```python
from build123d import *

# Parameters (mm, degrees)
SKETCH1_R               = 15
BOSS_EXTRUDE1_DEPTH     = 3.5
SKETCH2_R               = 2.121909517
SKETCH4_R               = 3.5
BOSS_EXTRUDE2_DEPTH     = 1
BOSS_EXTRUDE3_START     = 1
SKETCH5_R               = 3.5
BOSS_EXTRUDE3_DEPTH     = 1
CUT_EXTRUDE1_DEPTH      = 22.685248442
CUT_EXTRUDE1_DEPTH_BACK = 22.685248442
SKETCH3_R               = 2.5


with BuildPart() as part:
    # Sketch1 → Boss-Extrude1 (new body)
    with BuildSketch(Plane(origin=(0, 0, 0), x_dir=(1, 0, 0), z_dir=(0, 1, 0))):
        with Locations(Location((0, 0, 0), (0, 0, 270))):
            Circle(SKETCH1_R)
    extrude(amount=BOSS_EXTRUDE1_DEPTH)

    # Sketch2 → Cut-Revolve1 (revolve, cut)
    with BuildSketch(Plane(origin=(0, 0, 0), x_dir=(0, 0, -1), z_dir=(1, 0, 0)), mode=Mode.PRIVATE) as cut_revolve1_sk:
        with Locations((-16.2, 1.75)):
            Circle(SKETCH2_R)
    revolve(cut_revolve1_sk.sketch.rotate(Axis((0, 0, 0), (0, 1, 0)), 180), axis=Axis((0, 0, 0), (0, 1, 0)), mode=Mode.SUBTRACT)

    # Sketch4 → Boss-Extrude2 (add)
    with BuildSketch(Plane.XZ):
        with Locations(Location((0, 0, 0), (0, 0, 270))):
            Circle(SKETCH4_R)
    extrude(amount=BOSS_EXTRUDE2_DEPTH)

    # Sketch5 → Boss-Extrude3 (add)
    with BuildSketch(Plane(origin=(0, 3.5, 0), x_dir=(1, 0, 0), z_dir=(0, 1, 0)).offset(BOSS_EXTRUDE3_START)):
        with Locations(Location((0, 0, 0), (0, 0, 90))):
            Circle(SKETCH5_R)
    extrude(amount=-BOSS_EXTRUDE3_DEPTH)

    # Sketch3 → Cut-Extrude1 (cut, two sides: drawn at the far end of the back side and taken through both)
    with BuildSketch(Plane(origin=(0, 3.5, 0), x_dir=(1, 0, 0), z_dir=(0, 1, 0)).offset(-CUT_EXTRUDE1_DEPTH_BACK)):
        with Locations(Location((0, 0, 0), (0, 0, 270))):
            Circle(SKETCH3_R)
    extrude(amount=CUT_EXTRUDE1_DEPTH + CUT_EXTRUDE1_DEPTH_BACK, mode=Mode.SUBTRACT)


solid = part.part
```
Geometry check sheet. Reference: the model listing, model coordinates, mm. A direction names the side the tool comes from. Round coordinates to 2 decimals unless told otherwise and drop trailing zeros. Loops run counter-clockwise (first coordinate to the right, second up) from the corner with the lowest first, then second, coordinate; pieces in that order, holes last. Notation, with made-up numbers: (89.25, 15.25) - (143.25, 15.25) arc R34 cw to (143.25, 53.25) - close; hole circle Ø8 at (37.5, 30.5). An arc over 180 degrees is marked (long way). Write item = value, one per line. Start each with the question number.
1. Section check B-B on x = 0. Enter the section's corners in (y, z).
2. Set-up check for faces 1 (the face through (3.417, 4.007, 0.759)), 2 (the face through (-2, -1, -2)): record each of +Z, -Z, +X, -X, +Y, -Y from which the full face is reachable in a straight line by a thin tool's end or side.
3. Section check C-C on y = 0.45. Enter the section's corners in (x, z).
4. Thickness scan on line 1 (Y direction, x = 7.5, z = -11.5); line 2 (Z direction, x = 2, y = 0.2); line 3 (X direction, y = 1.1, z = 0). Record the ranges inside material, lowest first.
5. Depth check by flat-ended pin: pin 1 (3 mm diameter, centred on y = 1, z = 11, fed in from -X); pin 2 (6 mm diameter, centred on x = -5, z = -5, fed in from -Y); pin 3 (8 mm diameter, centred on x = 2.5, z = 10.5, fed in from +Y). Enter the tip coordinate at first touch or a pass-through.
6. Mould release check, pull along X, two halves, no side actions. Record for faces 3 (the face through (-3.417, -0.493, 0.759)), 4 (the face through (2, 4.5, -2)), 5 (the face through (-2.44, 1.71, -0.54)): released by +X, released by -X, zero draft, split by the parting line, or undercut.
7. Section check A-A on z = 0. Enter the section's corners in (x, y), then the cut area to 3 significant figures.
Working result:
q1.outline = (-1, -3.5) - (0, -3.5) - (0, -15) arc R2.12 cw to (3.5, -15) - (3.5, -3.5) - (4.5, -3.5) - (4.5, -2.5) - (-1, -2.5) - close; (-1, 2.5) - (4.5, 2.5) - (4.5, 3.5) - (3.5, 3.5) - (3.5, 15) arc R2.12 cw to (0, 15) - (0, 3.5) - (-1, 3.5) - close
q2.face_1 = +Y
q2.face_2 = +Z, -Z, +X, -X, -Y
q3.outline = circle Ø29.05 at (0, 0); hole circle Ø5 at (0, 0)
q4.line_1 = 0 to 3.5
q4.line_2 = -14.61 to -1.5, 1.5 to 14.61
q4.line_3 = -14.18 to -2.5, 2.5 to 14.18
q5.pin_1 = -11.28
q5.pin_2 = 0
q5.pin_3 = 3.5
q6.face_3 = split by the parting line
q6.face_4 = zero draft
q6.face_5 = undercut
q7.outline = (-15, 0) - (-3.5, 0) - (-3.5, -1) - (-2.5, -1) - (-2.5, 4.5) - (-3.5, 4.5) - (-3.5, 3.5) - (-15, 3.5) arc R2.12 cw to start; (2.5, -1) - (3.5, -1) - (3.5, 0) - (15, 0) arc R2.12 cw to (15, 3.5) - (3.5, 3.5) - (3.5, 4.5) - (2.5, 4.5) - close
q7.area = 87.0 mm^2
